Geometry: final body of the model. Coordinates: model frame, mm. A direction names the side the tool comes from. Coordinates: 2 decimals unless noted, no trailing zeros. Write each loop counter-clockwise with the first axis right and the second up, starting at its lowest first coordinate (ties: lowest second). Pieces come first, ordered by that corner, then holes. Notation, with made-up numbers: (10, 82) -> (54, 82) arc R12 ccw to (54, 98) -> close; hole circle Ø2 at (-40, 5.25). An arc over 180 degrees is marked (long way). One line per item, written item: value.
```python
from build123d import *

# Parameters (mm, degrees)
SKETCH1_R           = 1
BOSS_EXTRUDE1_DEPTH = 5
CUT_EXTRUDE1_DEPTH  = 13.599753478


with BuildPart() as part:
    # Sketch1 → Boss-Extrude1 (new body)
    with BuildSketch(Plane(origin=(0, 0, 0), x_dir=(0, 0, -1), z_dir=(1, 0, 0))):
        with BuildLine():
            ThreePointArc((0, 7.7), (1.5, 11.022875656), (3, 7.7))
            Line((3, 7.7), (3, 0))
            Line((3, 0), (0, 0))
            Line((0, 0), (0, 7.7))
        make_face()
        with Locations((1.5, 9.022875656)):
            Circle(SKETCH1_R, mode=Mode.SUBTRACT)
    extrude(amount=BOSS_EXTRUDE1_DEPTH)

    # Sketch2 → Cut-Extrude1 (cut, through all)
    with BuildSketch(Plane(origin=(0, 0, -3), x_dir=(-1, 0, 0), z_dir=(0, 0, -1))):
        with BuildLine():
            Line((-0.4, 5.1), (-0.4, 2.6))
            ThreePointArc((-0.4, 2.6), (-2, 1), (-3.6, 2.6))
            Line((-3.6, 2.6), (-3.6, 5.1))
            ThreePointArc((-3.6, 5.1), (-2, 6.7), (-0.4, 5.1))
        make_face()
    extrude(amount=-CUT_EXTRUDE1_DEPTH, mode=Mode.SUBTRACT)


solid = part.part
```
(1) Pull-direction query (Y, two-part tool) for faces 1 (the cylindrical face through (2.465, 10.014, -1.37)), 2 (the cylindrical face through (2.46, 11.02, -1.44)), 3 (the flat face through (4, 4, -3)); classes: released by +Y, released by -Y, zero draft, split by the parting line, or undercut.
Responses:
face 1: undercut
face 2: split by the parting line
face 3: zero draft
(2) Section D-D (z = -0.8). Return the cut outline in (x, y), then the cut area to 3 significant figures.
Responses:
outline: (0, 0) -> (5, 0) -> (5, 8.31) -> (0, 8.31) -> close; (0, 9.74) -> (5, 9.74) -> (5, 10.9) -> (0, 10.9) -> close; hole (0.4, 2.6) arc R1.6 ccw to (3.6, 2.6) -> (3.6, 5.1) arc R1.6 ccw to (0.4, 5.1) -> close
area: 31.3 mm2
(3) Section C-C (x = 2). Return the cut outline in (y, z).
Responses:
outline: (0, -3) -> (1, -3) -> (1, 0) -> (0, 0) -> close; (6.7, -3) -> (7.7, -3) arc R2 ccw (long way) to (7.7, 0) -> (6.7, 0) -> close; hole circle Ø2 at (9.02, -1.5)
(4) Reachability of faces 4 (the cylindrical face through (2, 1, -2)), 5 (the flat face through (4, 4, 0)), 6 (the flat face through (0, 6, -2)) from +Z, -Z, +X, -X, +Y, -Y: full face, straight path, thin tool, end or side. Return the list, or none.
Responses:
face 4: +Z, -Z
face 5: +Z, +X, -X, -Y
face 6: +Z, -Z, -X, +Y, -Y
(5) Line query: line 1 (Y direction, x = 3.3, z = -1.85); line 2 (X direction, y = 2.75, z = -1.05); line 3 (Y direction, x = 2.3, z = -1.5). Output: solid intervals per line, ascending. Write a range as [from, to].
Responses:
line 1: y = [0, 1.67], [6.03, 8.09], [9.96, 10.99]
line 2: x = [0, 0.4], [3.6, 5]
line 3: y = [0, 1.03], [6.67, 8.02], [10.02, 11.02]
(6) First-contact query: pin 1 (1.5 mm diameter, centred on x = 0.5, y = 8.5, fed in from -Z); pin 2 (1.5 mm diameter, centred on x = 2.5, y = 3, fed in from -Z); pin 3 (1.5 mm diameter, centred on x = 3.5, y = 3, fed in from +Z). Flat tips, straight axial feed; report the tip coordinate or a pass-through.
Responses:
pin 1: stops at z = -3.5
pin 2: passes through
pin 3: stops at z = 0
(7) Section B-B (y = 4.25). Return the cut outline in (x, z), then the cut area to 3 significant figures.
Responses:
outline: (0, -3) -> (0.4, -3) -> (0.4, 0) -> (0, 0) -> close; (3.6, -3) -> (5, -3) -> (5, 0) -> (3.6, 0) -> close
area: 5.40 mm2
(8) Section A-A (z = -1.5). Return the cut outline in (x, y), then the cut area to 3 significant figures.
Responses:
outline: (0, 0) -> (5, 0) -> (5, 8.02) -> (0, 8.02) -> close; (0, 10.02) -> (5, 10.02) -> (5, 11.02) -> (0, 11.02) -> close; hole (0.4, 2.6) arc R1.6 ccw to (3.6, 2.6) -> (3.6, 5.1) arc R1.6 ccw to (0.4, 5.1) -> close
area: 29.1 mm2
